Could you check a few things on this drawing? It's one solid part, dimensions in mm from its lowest x, y, z. Give positions to 0.01 mm unless a question says otherwise; leave off trailing zeros. Write each loop counter-clockwise with the first axis right and the second up, starting at its lowest first coordinate (ties: lowest second). Pieces come first, ordered by that corner, then holes. Notation, with made-up numbers: (6, 16) -> (18, 16) arc R20 ccw to (18, 24) -> close; hole circle Ø8 at (64, 19.5). An arc over 180 degrees is marked (long way). Use CSV: the item, a comma, the result in double quotes. Start each with the question number.
(1) Suppose I cut it at A-A on z = 6.35. List the corners of the cut face in (x, y) for me.
(2) For pin 1 Ø3 at (x, z) = (172.5, 124.5) entering from +Y; pin 2 Ø5 at (x, z) = (264, 211) entering from -Y, each with a flat end and sliding along its axis, tell me the tip position at first contact or that it passes through.
(3) I need wall thicknesses on L1, parallel to Y at x = 262.5, z = 30.5. Which ranges of the line are inside material? Lowest first, please. Write a range as [from, to].
(4) Suppose I cut it at B-B on x = 247. List the corners of the cut face in (y, z) for me.
(5) Suppose I cut it at C-C on z = 222. List the corners of the cut face in (x, y) for me.
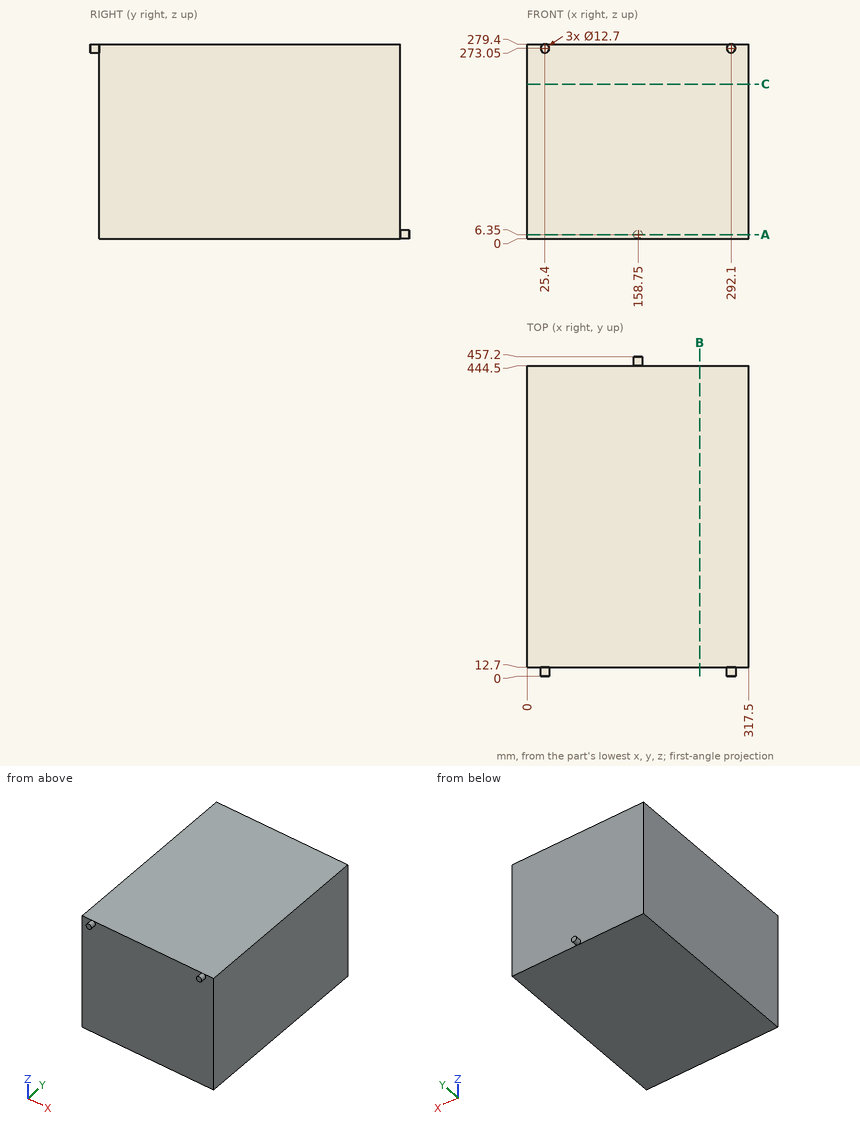
Geometry says:
1,outline,"(0, 12.7) -> (317.5, 12.7) -> (317.5, 444.5) -> (165.1, 444.5) -> (165.1, 457.2) -> (152.4, 457.2) -> (152.4, 444.5) -> (0, 444.5) -> close"
2,pin 1,"y = 444.5"
2,pin 2,"y = 12.7"
3,L1,"[12.7, 444.5]"
4,outline,"(12.7, 0) -> (444.5, 0) -> (444.5, 279.4) -> (12.7, 279.4) -> close"
5,outline,"(0, 12.7) -> (317.5, 12.7) -> (317.5, 444.5) -> (0, 444.5) -> close"
